from build123d import *

# Parameters (mm, degrees)
F0_W     = 76
F0_H     = 57.5
F0_R     = 2
F0_W_2   = 48
F0_H_2   = 27.5
F1_DEPTH = 1
F2_R     = 10
F3_SIZE  = 5


with BuildPart() as f1:
    # F0 (on Top) → F1 (new body)
    with BuildSketch(Plane.XY):
        Rectangle(F0_W, F0_H)
        with Locations((0, -20.25)):
            Circle(F0_R, mode=Mode.SUBTRACT)
        Rectangle(F0_W_2, F0_H_2, mode=Mode.SUBTRACT)
        with Locations((0, 19.75)):
            Circle(F0_R, mode=Mode.SUBTRACT)
    extrude(amount=F1_DEPTH)

    # F2
    f2_edges = [f1.edges().sort_by_distance(p)[0] for p in [
        (-38, 28.75, 0.5),
        (-38, -28.75, 0.5),
        (38, 28.75, 0.5),
        (38, -28.75, 0.5),
    ]]
    fillet(f2_edges, radius=F2_R)

    # F3
    f3_edges = [f1.edges().sort_by_distance(p)[0] for p in [
        (24, 13.75, 0.5),
        (24, -13.75, 0.5),
    ]]
    chamfer(f3_edges, length=F3_SIZE)


solid = f1.part
Part model, mm, in its own coordinate system. A direction names the side the tool comes from. Give positions to 0.01 mm unless a question says otherwise; leave off trailing zeros. Loops run counter-clockwise (first coordinate to the right, second up) from the corner with the lowest first, then second, coordinate; pieces in that order, holes last. Notation, with made-up numbers: (65.25, -2.5) -> (78.25, -2.5) arc R10 ccw to (78.25, 6.5) -> close; hole circle Ø11 at (9.25, -23.75). An arc over 180 degrees is marked (long way). Write each question's results on one line, items separated by ' | '. Start each with the question number.
Q1. Band-saw the part on B-B on x = 8. List the corners of the cut face in (y, z), plus the area to 3 significant figures.
Q2. Wall check: L1, parallel to Y at x = 0, z = 0.65; L2, parallel to Y at x = 5, z = 0.2; L3, parallel to X at y = 2, z = 0.35. Give the ranges that are in metal, low to high.
Q3. Pin check, flat tip, straight feed: P1, Ø3.5, axis at x = 0, y = -20.25, coming from the -Z side. Stop position of the tip, or through.
Q4. Band-saw the part on C-C on x = 0. List the corners of the cut face in (y, z).
Q5. Band-saw the part on D-D on z = 0.4. List the corners of the cut face in (x, y).
Q6. Which spindle directions (+Z, -Z, +X, -X, +Y, -Y) get a long thin tool onto all of the face, cutting with end or side? Do faces 4 (the face through (-9, 20, 1)), 5 (the face through (21.465, 11.285, 0.493)). Say none if no direction does.
Q7. Pull direction X, two halves, no side cores. Call faces 1 (the face through (21.535, -11.215, 0.493)), 2 (the face through (-35.15, -25.74, 0.51)), 3 (the face through (34.99, 25.9, 0.51)): +X half, -X half, draft (parallel to the pull), parting line (faces both ways), or undercut.
Q8. Band-saw the part on A-A on y = 6. List the corners of the cut face in (x, z).
Results are:
1) outline: (-28.75, 0) -> (-13.75, 0) -> (-13.75, 1) -> (-28.75, 1) -> close; (13.75, 0) -> (28.75, 0) -> (28.75, 1) -> (13.75, 1) -> close | area: 30.0 mm²
2) L1: y = -28.75 to -22.25, -18.25 to -13.75, 13.75 to 17.75, 21.75 to 28.75 | L2: y = -28.75 to -13.75, 13.75 to 28.75 | L3: x = -38 to -24, 24 to 38
3) P1: passes through
4) outline: (-28.75, 0) -> (-22.25, 0) -> (-22.25, 1) -> (-28.75, 1) -> close; (-18.25, 0) -> (-13.75, 0) -> (-13.75, 1) -> (-18.25, 1) -> close; (13.75, 0) -> (17.75, 0) -> (17.75, 1) -> (13.75, 1) -> close; (21.75, 0) -> (28.75, 0) -> (28.75, 1) -> (21.75, 1) -> close
5) outline: (-38, -18.75) arc R10 ccw to (-28, -28.75) -> (28, -28.75) arc R10 ccw to (38, -18.75) -> (38, 18.75) arc R10 ccw to (28, 28.75) -> (-28, 28.75) arc R10 ccw to (-38, 18.75) -> close; hole (-24, -13.75) -> (19, -13.75) -> (24, -8.75) -> (24, 8.75) -> (19, 13.75) -> (-24, 13.75) -> close; hole circle Ø4 at (0, -20.25); hole circle Ø4 at (0, 19.75)
6) face 4: +Z, +X, -X, +Y, -Y | face 5: +Z, -Z
7) face 1: undercut | face 2: -X half | face 3: +X half
8) outline: (-38, 0) -> (-24, 0) -> (-24, 1) -> (-38, 1) -> close; (24, 0) -> (38, 0) -> (38, 1) -> (24, 1) -> close
